For this review, take the finished solid that the model builds, in its own axes (mm). Round coordinates to 2 decimals unless told otherwise and drop trailing zeros. Loops run counter-clockwise (first coordinate to the right, second up) from the corner with the lowest first, then second, coordinate; pieces in that order, holes last. Notation, with made-up numbers: (-16, -9.5) -> (37, -9.5) arc R24 cw to (37, 20.5) -> close; hole circle Ø6 at (43.5, 28). An arc over 180 degrees is marked (long way). Write each question's results on one line, items separated by ' | '.
```python
from build123d import *

# Parameters (mm, degrees)
BOSS_EXTRUDE1_DEPTH   = 28.5
M6_TAPPED_HOLE1_D     = 5
M6_TAPPED_HOLE1_DEPTH = 6
M6_TAPPED_HOLE1_TIP   = 1.502151548
M6_TAPPED_HOLE2_D     = 5
M6_TAPPED_HOLE2_DEPTH = 8
M6_TAPPED_HOLE2_TIP   = 1.502151548
SKETCH6_R             = 2.5
CUT_EXTRUDE2_DEPTH    = 29.5
SKETCH5_R             = 1.55
CUT_EXTRUDE1_DEPTH    = 13.7


with BuildPart() as part:
    # Sketch1 → Boss-Extrude1 (new body)
    with BuildSketch(Plane.XY):
        Polygon((11.849261314, 3.175), (6.35, 0), (31.75, 0), (26.250738686, 3.175), (26.250738686, 9.525), (31.75, 12.7), (6.35, 12.7), (11.849261314, 9.525), align=None)
        Polygon((0.850738686, 9.525), (0.850738686, 3.175), (6.35, 0), (11.849261314, 3.175), (11.849261314, 9.525), (6.35, 12.7), align=None)
        Polygon((26.250738686, 9.525), (26.250738686, 3.175), (31.75, 0), (37.249261314, 3.175), (37.249261314, 9.525), (31.75, 12.7), align=None)
    extrude(amount=-BOSS_EXTRUDE1_DEPTH)

    # M6 Tapped Hole1
    with Locations(Plane.XY):
        with Locations((19.05, 6.35), (31.75, 6.35), (6.35, 6.35)):
            Hole(M6_TAPPED_HOLE1_D / 2, depth=M6_TAPPED_HOLE1_DEPTH)
            with Locations((0, 0, -(M6_TAPPED_HOLE1_DEPTH + M6_TAPPED_HOLE1_TIP / 2))):  # 118° drill point
                Cone(0, M6_TAPPED_HOLE1_D / 2, M6_TAPPED_HOLE1_TIP, mode=Mode.SUBTRACT)

    # M6 Tapped Hole2
    with Locations(Plane(origin=(0, 0, -28.5), x_dir=(-1, 0, 0), z_dir=(0, 0, -1))):
        with Locations((-31.75, 6.35), (-19.05, 6.35), (-6.35, 6.35)):
            Hole(M6_TAPPED_HOLE2_D / 2, depth=M6_TAPPED_HOLE2_DEPTH)
            with Locations((0, 0, -(M6_TAPPED_HOLE2_DEPTH + M6_TAPPED_HOLE2_TIP / 2))):  # 118° drill point
                Cone(0, M6_TAPPED_HOLE2_D / 2, M6_TAPPED_HOLE2_TIP, mode=Mode.SUBTRACT)

    # Sketch6 → Cut-Extrude2 (cut, through all)
    with BuildSketch(Plane.XY):
        with Locations((6.35, 6.35)):
            Circle(SKETCH6_R)
        with Locations((19.05, 6.35)):
            Circle(SKETCH6_R)
        with Locations((31.75, 6.35)):
            Circle(SKETCH6_R)
    extrude(amount=-CUT_EXTRUDE2_DEPTH, mode=Mode.SUBTRACT)

    # Sketch5 → Cut-Extrude1 (cut, through all)
    with BuildSketch(Plane(origin=(0, 12.7, 0), x_dir=(1, 0, 0), z_dir=(0, 1, 0))):
        with Locations((12.7, 23.5)):
            Circle(SKETCH5_R)
        with Locations((25.4, 23.5)):
            Circle(SKETCH5_R)
        with Locations((25.4, 5)):
            Circle(SKETCH5_R)
        with Locations((12.7, 5)):
            Circle(SKETCH5_R)
    extrude(amount=-CUT_EXTRUDE1_DEPTH, mode=Mode.SUBTRACT)


solid = part.part
```
1. To check wall thickness, follow probe 1 along X at (y, z) = (2.75, -22.5); probe 2 along X at (y, z) = (8.25, -23.5); probe 3 along Z at (x, y) = (26, 3.5). State the ranges of each line that lie inside material, in increasing order.
Values found:
probe 1: x = 1.59 to 11.52, 13.88 to 24.22, 26.58 to 36.51 | probe 2: x = 0.85 to 4.73, 7.97 to 11.15, 14.25 to 17.43, 20.67 to 23.85, 26.95 to 30.13, 33.37 to 37.25 | probe 3: z = -28.5 to -24.93, -22.07 to -6.43, -3.57 to 0
2. Draft analysis for pull direction X (two halves, no side actions). For faces 1 (the face through (3.639, 11.135, -14.05)), 2 (the face through (12.498, 6.439, -25.037)), 3 (the face through (19, 0, -14)), 4 (the face through (34.461, 1.565, -14.05)), state which applies: released by +X, released by -X, zero draft, split by the parting line, or undercut.
Values found:
face 1: released by -X | face 2: undercut | face 3: zero draft | face 4: released by +X
3. Consider section A-A (z = -19). State the section outline as (x, y) points (3 decimals).
Values found:
outline: (0.851, 3.175) -> (6.35, 0) -> (31.75, 0) -> (37.249, 3.175) -> (37.249, 9.525) -> (31.75, 12.7) -> (6.35, 12.7) -> (0.851, 9.525) -> close; hole circle Ø5 at (6.35, 6.35); hole circle Ø5 at (19.05, 6.35); hole circle Ø5 at (31.75, 6.35)
4. Consider section B-B (y = 4.5). State the section outline as (x, z) points.
Values found:
outline: (0.85, -28.5) -> (4.67, -28.5) -> (4.67, 0) -> (0.85, 0) -> close; (8.03, -28.5) -> (17.37, -28.5) -> (17.37, 0) -> (8.03, 0) -> close; (20.73, -28.5) -> (30.07, -28.5) -> (30.07, 0) -> (20.73, 0) -> close; (33.43, -28.5) -> (37.25, -28.5) -> (37.25, 0) -> (33.43, 0) -> close; hole circle Ø3.1 at (12.7, -23.5); hole circle Ø3.1 at (12.7, -5); hole circle Ø3.1 at (25.4, -23.5); hole circle Ø3.1 at (25.4, -5)
5. For pin 1 (5 mm diameter, centred on x = 12.7, z = -5, fed in from +Y); pin 2 (3 mm diameter, centred on x = 19.05, y = 6.35, fed in from -Z), all flat-tipped, find the tip position at first contact; note any pin that passes through.
Values found:
pin 1: stops at y = 12.7 | pin 2: passes through
6. Consider section C-C (x = 25.4). State the section outline as (y, z) points.
Values found:
outline: (0, -28.5) -> (12.7, -28.5) -> (12.7, -25.05) -> (0, -25.05) -> close; (0, -21.95) -> (12.7, -21.95) -> (12.7, -6.55) -> (0, -6.55) -> close; (0, -3.45) -> (12.7, -3.45) -> (12.7, 0) -> (0, 0) -> close
7. Consider section D-D (x = 19.05). State the section outline as (y, z) points.
Values found:
outline: (0, -28.5) -> (3.85, -28.5) -> (3.85, 0) -> (0, 0) -> close; (8.85, -28.5) -> (12.7, -28.5) -> (12.7, 0) -> (8.85, 0) -> close
